```python
from build123d import *

# Parameters (mm, degrees)
SKETCH1_R           = 9
SKETCH1_R_2         = 4
BOSS_EXTRUDE1_DEPTH = 1
SKETCH2_R           = 8
SKETCH2_R_2         = 4
BOSS_EXTRUDE2_DEPTH = 4
SKETCH3_R           = 6.75
SKETCH3_R_2         = 5.25
CUT_EXTRUDE1_DEPTH  = 0.6
CUT_EXTRUDE2_START  = -0.6
SKETCH4_R           = 6.75
SKETCH4_R_2         = 5.25
CUT_EXTRUDE2_DEPTH  = 0.6


with BuildPart() as part:
    # Sketch1 → Boss-Extrude1 (new body)
    with BuildSketch(Plane(origin=(0, 0, 0), x_dir=(1, 0, 0), z_dir=(0, 1, 0))):
        with Locations(Location((0, 0, 0), (0, 0, 270))):
            Circle(SKETCH1_R)
        with Locations(Location((0, 0, 0), (0, 0, 270))):
            Circle(SKETCH1_R_2, mode=Mode.SUBTRACT)
    extrude(amount=BOSS_EXTRUDE1_DEPTH)

    # Sketch2 → Boss-Extrude2 (add)
    with BuildSketch(Plane(origin=(0, 1, 0), x_dir=(1, 0, 0), z_dir=(0, 1, 0))):
        with Locations(Location((0, 0, 0), (0, 0, 270))):
            Circle(SKETCH2_R)
        with Locations(Location((0, 0, 0), (0, 0, 270))):
            Circle(SKETCH2_R_2, mode=Mode.SUBTRACT)
    extrude(amount=BOSS_EXTRUDE2_DEPTH)

    # Sketch3 → Cut-Extrude1 (cut)
    with BuildSketch(Plane(origin=(0, 5, 0), x_dir=(1, 0, 0), z_dir=(0, 1, 0))):
        with Locations(Location((0, 0, 0), (0, 0, 270))):
            Circle(SKETCH3_R)
        with Locations(Location((0, 0, 0), (0, 0, 270))):
            Circle(SKETCH3_R_2, mode=Mode.SUBTRACT)
    extrude(amount=-CUT_EXTRUDE1_DEPTH, mode=Mode.SUBTRACT)

    # Sketch4 → Cut-Extrude2 (cut)
    with BuildSketch(Plane(origin=(0, 0, 0), x_dir=(-1, 0, 0), z_dir=(0, -1, 0)).offset(CUT_EXTRUDE2_START)):
        with Locations(Location((0, 0, 0), (0, 0, 270))):
            Circle(SKETCH4_R)
        with Locations(Location((0, 0, 0), (0, 0, 270))):
            Circle(SKETCH4_R_2, mode=Mode.SUBTRACT)
    extrude(amount=CUT_EXTRUDE2_DEPTH, mode=Mode.SUBTRACT)


solid = part.part
```
Can you work these out from the model? Positions are in its coordinate system, mm. A direction names the side the tool comes from. Coordinates: 2 decimals unless noted, no trailing zeros. Loops run counter-clockwise (first coordinate to the right, second up) from the corner with the lowest first, then second, coordinate; pieces in that order, holes last. Notation, with made-up numbers: (74, 22) - (133, 22) arc R18 cw to (133, 50) - close; hole circle Ø9 at (70, -27). An arc over 180 degrees is marked (long way). Answer as CSV lines item,"result". Start each with the question number.
1) For pin 1 (5 mm diameter, centred on x = 2, z = 1, fed in from -Y); pin 2 (1.5 mm diameter, centred on x = 6.5, y = 2, fed in from -Z); pin 3 (1 mm diameter, centred on x = -5.5, y = 3, fed in from -Z) (3 decimals); pin 4 (1 mm diameter, centred on x = 7, y = 4.5, fed in from +Z), each with a flat end and sliding along its axis, tell me the tip position at first contact or that it passes through.
2) Suppose I cut it at B-B (x = 0). Please give me the cut outline in (y, z), plus the area to 3 significant figures.
3) Suppose I cut it at A-A (z = 0). Please give me the cut outline in (x, y), plus the area to 3 significant figures.
4) Which directions (+Z, -Z, +X, -X, +Y, -Y) give clear straight access to the entire face, cutting with the end or side of a thin tool? Please do faces 1 (the flat face through (-5.5, 4.4, 0)), 2 (the cylindrical face through (6.59, 0.3, -1.46)), 3 (the flat face through (-2, 5, -4)).
5) Suppose I cut it at C-C (y = 4). Please give me the cut outline in (x, z), plus the area to 3 significant figures.
6) Thinking about a two-plate mould opening in Z: for faces 4 (the cylindrical face through (-6.59, 4.7, -1.46)), 5 (the cylindrical face through (-7.81, 2.97, -1.73)), 6 (the flat face through (-2, 0, -4)), which applies, pulls with the +Z half, pulls with the -Z half, needs draft (parallel to the pull), parting line crosses it, or undercut?
7) I need wall thicknesses on line 1 (X direction, y = 4.8, z = 0); line 2 (X direction, y = 0.55, z = 0); line 3 (Z direction, x = 3, y = 4.65). Which ranges of each line are inside material? Lowest first, please. Write a range as from..to.
8) Suppose I cut it at D-D (z = -6.5). Please give me the cut outline in (x, y).
Check result:
1,pin 1,"stops at y = 0"
1,pin 2,"stops at z = -5.56"
1,pin 3,"stops at z = -6.245"
1,pin 4,"stops at z = 4.66"
2,outline,"(0, -9) - (1, -9) - (1, -8) - (5, -8) - (5, -6.75) - (4.4, -6.75) - (4.4, -5.25) - (5, -5.25) - (5, -4) - (0, -4) - (0, -5.25) - (0.6, -5.25) - (0.6, -6.75) - (0, -6.75) - close; (0, 4) - (5, 4) - (5, 5.25) - (4.4, 5.25) - (4.4, 6.75) - (5, 6.75) - (5, 8) - (1, 8) - (1, 9) - (0, 9) - (0, 6.75) - (0.6, 6.75) - (0.6, 5.25) - (0, 5.25) - close"
2,area,"38.4 mm²"
3,outline,"(-9, 0) - (-6.75, 0) - (-6.75, 0.6) - (-5.25, 0.6) - (-5.25, 0) - (-4, 0) - (-4, 5) - (-5.25, 5) - (-5.25, 4.4) - (-6.75, 4.4) - (-6.75, 5) - (-8, 5) - (-8, 1) - (-9, 1) - close; (4, 0) - (5.25, 0) - (5.25, 0.6) - (6.75, 0.6) - (6.75, 0) - (9, 0) - (9, 1) - (8, 1) - (8, 5) - (6.75, 5) - (6.75, 4.4) - (5.25, 4.4) - (5.25, 5) - (4, 5) - close"
3,area,"38.4 mm²"
4,face 1,"+Y"
4,face 2,"-Y"
4,face 3,"+Z, -Z, +X, -X, +Y"
5,outline,"circle Ø16 at (0, 0); hole circle Ø8 at (0, 0)"
5,area,"151 mm²"
6,face 4,"undercut"
6,face 5,"parting line crosses it"
6,face 6,"needs draft"
7,line 1,"x = -8..-6.75, -5.25..-4, 4..5.25, 6.75..8"
7,line 2,"x = -9..-6.75, -5.25..-4, 4..5.25, 6.75..9"
7,line 3,"z = -7.42..-6.05, -4.31..-2.65, 2.65..4.31, 6.05..7.42"
8,outline,"(-6.22, 0) - (-1.82, 0) - (-1.82, 0.6) - (1.82, 0.6) - (1.82, 0) - (6.22, 0) - (6.22, 1) - (4.66, 1) - (4.66, 5) - (1.82, 5) - (1.82, 4.4) - (-1.82, 4.4) - (-1.82, 5) - (-4.66, 5) - (-4.66, 1) - (-6.22, 1) - close"
